The listing builds one solid part. Answer for the finished solid, in the listing's coordinates (mm). Face numbers are marked on the shaded views. A direction names the side the tool comes from. Give positions to 0.01 mm unless a question says otherwise; leave off trailing zeros. Loops run counter-clockwise (first coordinate to the right, second up) from the corner with the lowest first, then second, coordinate; pieces in that order, holes last. Notation, with made-up numbers: M -0.5,2 L 45.5,2 A25 ccw 45.5,16 Z; hole C 41.25,-13.75 d1. An arc over 180 degrees is marked long. Return JSON: item names as keys, results as strings.
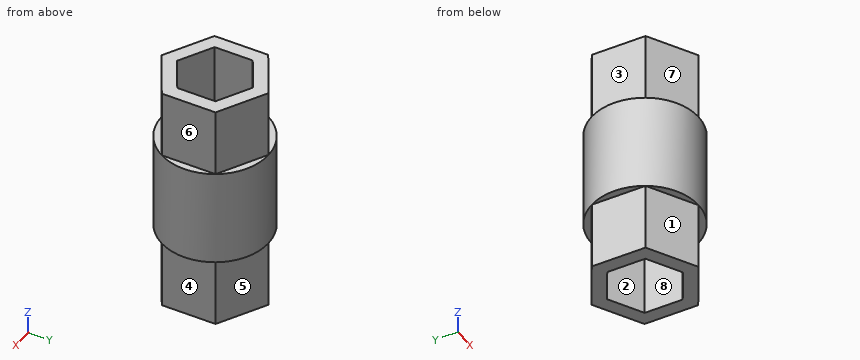
from build123d import *

# Parameters (mm, degrees)
SKETCH1_R           = 11
SKETCH1_R_2         = 6.4
BOSS_EXTRUDE1_DEPTH = 10
BOSS_EXTRUDE2_DEPTH = 24
CUT_EXTRUDE3_DEPTH  = 49


with BuildPart() as part:
    # Sketch1 → Boss-Extrude1 (new body, symmetric)
    with BuildSketch(Plane.XY):
        Circle(SKETCH1_R)
        Circle(SKETCH1_R_2, mode=Mode.SUBTRACT)
    extrude(amount=BOSS_EXTRUDE1_DEPTH, both=True)

    # Sketch1_3 → Boss-Extrude2 (add, symmetric)
    with BuildSketch(Plane.XY):
        Polygon((0, -11), (9.526279442, -5.5), (9.526279442, 5.5), (0, 11), (-9.526279442, 5.5), (-9.526279442, -5.5), align=None)
    extrude(amount=BOSS_EXTRUDE2_DEPTH, both=True)

    # Sketch2 → Cut-Extrude3 (cut, through all)
    with BuildSketch(Plane.XY.offset(24)):
        Polygon((0, -7.8), (6.75499815, -3.9), (6.75499815, 3.9), (0, 7.8), (-6.75499815, 3.9), (-6.75499815, -3.9), align=None)
    extrude(amount=-CUT_EXTRUDE3_DEPTH, mode=Mode.SUBTRACT)


solid = part.part
(1) Determine the mould class of the marked faces 6, 7 and 8 for opening direction X: released by +X, released by -X, zero draft, split by the parting line, or undercut.
Values follow:
{"face 6": "released by +X", "face 7": "released by -X", "face 8": "undercut"}
(2) Straight lines are drawn through the part: line 1 along X through (y, z) = (-0.25, 15.5) (3 decimals); line 2 along X through (y, z) = (-4.25, 20.5); line 3 along Y through (x, z) = (7.75, -8.5). For each, find the intervals that lie inside material, in ascending order.
Values follow:
{"line 1": "-9.526 to -6.755, 6.755 to 9.526", "line 2": "-9.53 to -6.15, 6.15 to 9.53", "line 3": "-7.81 to 7.81"}
(3) The part is cut by section C-C (x = 4.5). Determine the outline of the cut face in (y, z).
Values follow:
{"outline": "M -10.04,-10 L -8.4,-10 L -8.4,-24 L -5.2,-24 L -5.2,24 L -8.4,24 L -8.4,10 L -10.04,10 Z; M 5.2,-24 L 8.4,-24 L 8.4,-10 L 10.04,-10 L 10.04,10 L 8.4,10 L 8.4,24 L 5.2,24 Z"}
(4) The part is cut by section B-B (y = 0). Determine the outline of the cut face in (x, z) (3 decimals), and give its area (3 significant figures).
Values follow:
{"outline": "M -11,-10 L -9.526,-10 L -9.526,-24 L -6.755,-24 L -6.755,24 L -9.526,24 L -9.526,10 L -11,10 Z; M 6.755,-24 L 9.526,-24 L 9.526,-10 L 11,-10 L 11,10 L 9.526,10 L 9.526,24 L 6.755,24 Z", "area": "325 mm²"}
(5) The part is cut by section D-D (z = -18.5). Determine the outline of the cut face in (x, y) (3 decimals), and give its area (3 significant figures).
Values follow:
{"outline": "M -9.526,-5.5 L 0,-11 L 9.526,-5.5 L 9.526,5.5 L 0,11 L -9.526,5.5 Z; hole M -6.755,-3.9 L 0,-7.8 L 6.755,-3.9 L 6.755,3.9 L 0,7.8 L -6.755,3.9 Z", "area": "156 mm²"}
(6) Given pin 1 (3.5 mm diameter, centred on y = -2.5, z = -20, fed in from -X); pin 2 (5 mm diameter, centred on x = -4.5, z = 10, fed in from +Y); pin 3 (1.7 mm diameter, centred on x = -6.5, y = -9.5, fed in from +Z); pin 4 (2 mm diameter, centred on y = -1, z = 2, fed in from +X), each flat-ended and moving along its own axis, determine where each tip first touches the part or whether it passes through.
Values follow:
{"pin 1": "x = -9.53", "pin 2": "y = 10.82", "pin 3": "z = 10", "pin 4": "x = 11"}
(7) The part is cut by section A-A (z = 6). Determine the outline of the cut face in (x, y) (3 decimals).
Values follow:
{"outline": "C 0,0 d22; hole M -6.755,-3.9 L 0,-7.8 L 6.755,-3.9 L 6.755,3.9 L 0,7.8 L -6.755,3.9 Z"}
(8) A tool of negligible diameter and unlimited length cuts with its end or side. For the marked faces 1, 2, 3, 4 and 5, from which of +Z, -Z, +X, -X, +Y, -Y can it reach the whole face along a straight path? Write none if from no direction.
Values follow:
{"face 1": "-Z, -X, -Y", "face 2": "+Z, -Z", "face 3": "+Z, -X, +Y, -Y", "face 4": "-Z, +X, +Y, -Y", "face 5": "-Z, +X, +Y"}
